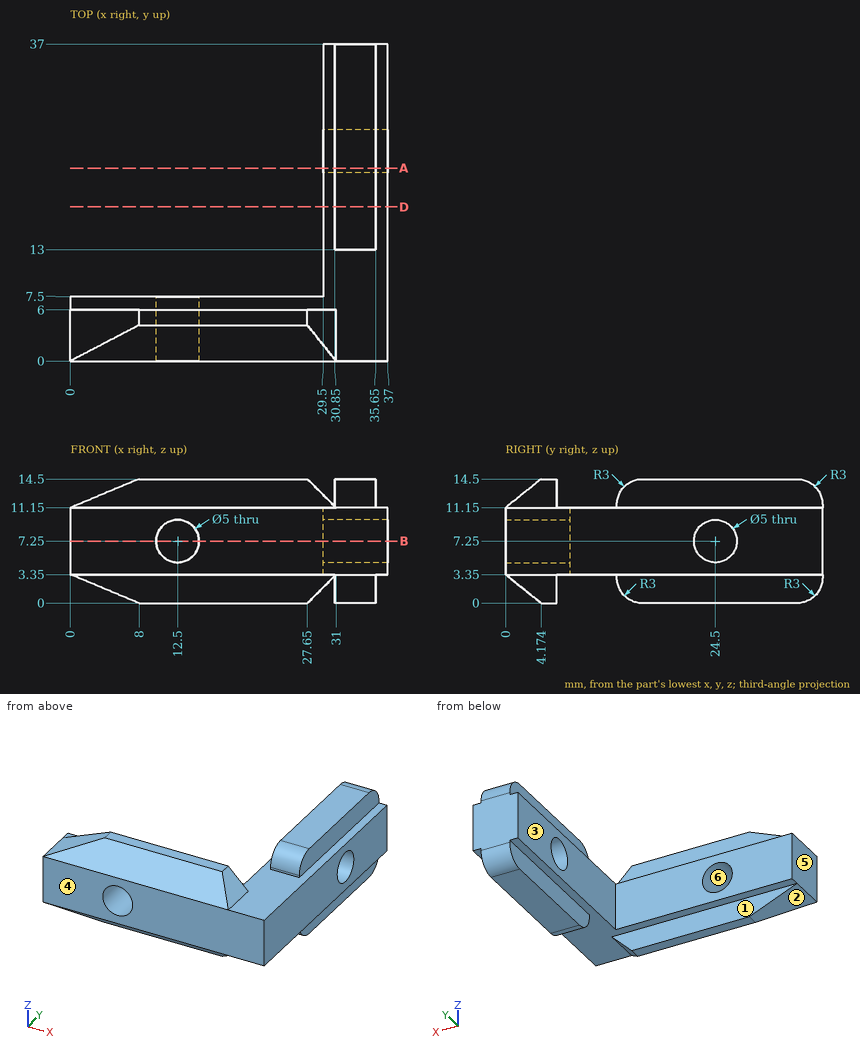
Source: three-view drawing plus pictorial views. Frame: mm from the lowest corner of the part. A direction names the side the tool comes from. Round coordinates to 2 decimals unless told otherwise and drop trailing zeros. Order: outer loops, then holes, each group sorted by start corner. A loop starts at its lowest first (then second) coordinate and runs counter-clockwise, first axis right, second up. Notation, with made-up numbers: (-38.75, 23) -> (-19.75, 23) arc R21 ccw to (-19.75, 50) -> close; hole circle Ø9 at (-6, 5). An arc over 180 degrees is marked (long way). Use CSV: the item, a comma, the result in double quotes. Start each with the question number.
1) Section D-D (y = 18). Return the cut outline in (x, z).
2) Set-up query: the marked faces 1, 2 and 3. Return all of +Z, -Z, +X, -X, +Y, -Y with unobstructed straight access to the full face (end or side cutting, diameter ignored); none if empty.
3) Section A-A (y = 22.5). Return the cut outline in (x, z).
4) Material intervals for line 1 along X through (y, z) = (2.5, 7.25); line 2 along Y through (x, z) = (34.5, 7.25); line 3 along Y through (x, z) = (27, 3.75), sorted ascending. Write a range as from..to.
5) First-contact query: pin 1 Ø1.7 at (y, z) = (21, 2) entering from -X; pin 2 Ø1 at (x, z) = (13, 9.5) entering from +Y; pin 3 Ø1.7 at (y, z) = (25, 12.5) entering from +X; pin 4 Ø6.5 at (x, z) = (12.5, 7.25) entering from -Y. Flat tips, straight axial feed; report the tip coordinate or a pass-through.
6) Section B-B (z = 7.25). Return the cut outline in (x, y), and give its area (3 significant figures).
7) Draft query along X for the marked faces 4, 5 and 6. Return one class per face: +X half, -X half, draft (parallel to the pull), parting line (faces both ways), or undercut.
Returned:
1,outline,"(29.5, 3.35) -> (30.85, 3.35) -> (30.85, 0) -> (35.65, 0) -> (35.65, 3.35) -> (37, 3.35) -> (37, 11.15) -> (35.65, 11.15) -> (35.65, 14.5) -> (30.85, 14.5) -> (30.85, 11.15) -> (29.5, 11.15) -> close"
2,face 1,"-Z, +X, -X, +Y"
2,face 2,"-Z, -X, +Y, -Y"
2,face 3,"+Z, -Z, -X, +Y"
3,outline,"(29.5, 3.35) -> (30.85, 3.35) -> (30.85, 0) -> (35.65, 0) -> (35.65, 3.35) -> (37, 3.35) -> (37, 5.75) -> (29.5, 5.75) -> close; (29.5, 8.75) -> (37, 8.75) -> (37, 11.15) -> (35.65, 11.15) -> (35.65, 14.5) -> (30.85, 14.5) -> (30.85, 11.15) -> (29.5, 11.15) -> close"
4,line 1,"x = 0..10, 15..37"
4,line 2,"y = 0..22, 27..37"
4,line 3,"y = 0..7.5"
5,pin 1,"stops at x = 30.85"
5,pin 2,"stops at y = 7.5"
5,pin 3,"stops at x = 35.65"
5,pin 4,"stops at y = 0"
6,outline,"(0, 0) -> (10, 0) -> (10, 7.5) -> (0, 7.5) -> close; (15, 0) -> (37, 0) -> (37, 22) -> (29.5, 22) -> (29.5, 7.5) -> (15, 7.5) -> close; (29.5, 27) -> (37, 27) -> (37, 37) -> (29.5, 37) -> close"
6,area,"424 mm²"
7,face 4,"draft"
7,face 5,"-X half"
7,face 6,"undercut"
